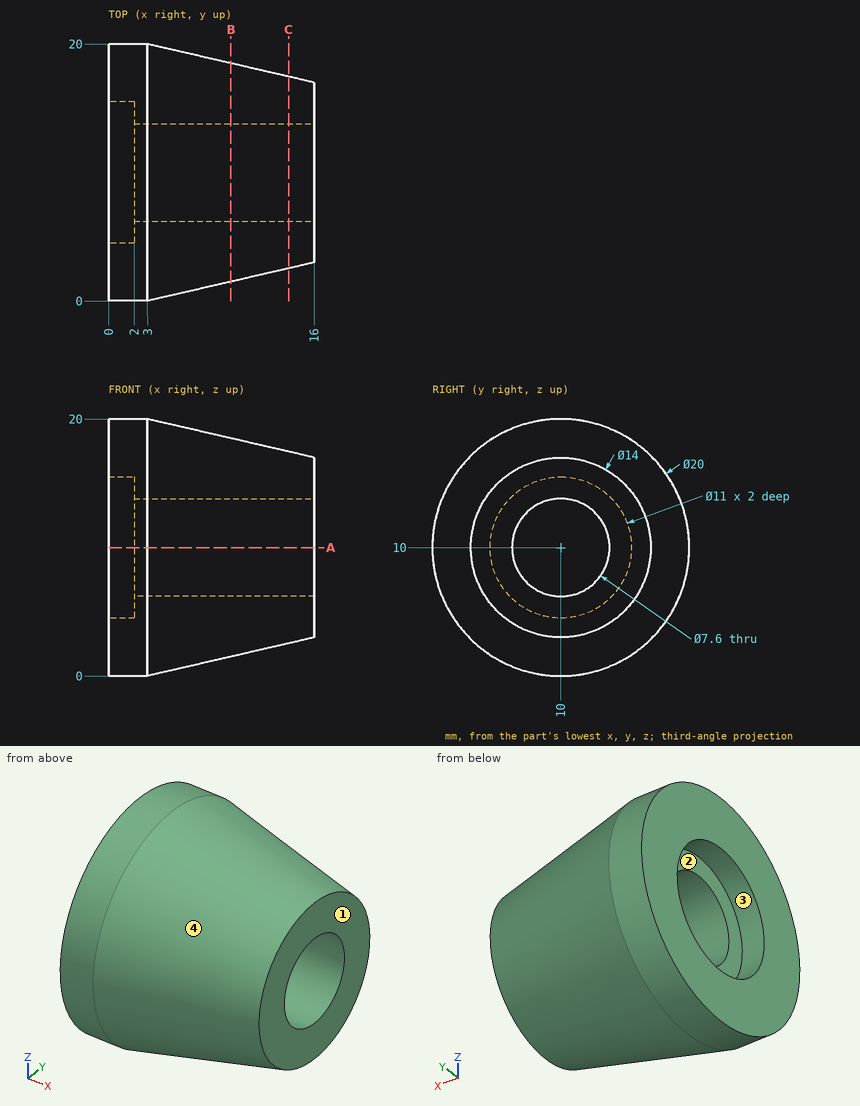
Geometry check sheet. Reference: drawing and pictorial views, mm from the part's lowest x, y, z. Give positions to 0.01 mm unless a question says otherwise; leave off trailing zeros. Write each loop counter-clockwise with the first axis right and the second up, starting at its lowest first coordinate (ties: lowest second). Pieces come first, ordered by that corner, then holes. Notation, with made-up numbers: M -8,58 L 24,58 A23 cw 24,78 Z; hole C 29.5,76.5 d5. An arc over 180 degrees is marked long. Answer as CSV lines item,"result". Start each with the question number.
Q1. Release check for a two-part mould opening along Y. For the marked faces 1, 2, 3 and 4 record: pulls with the +Y half, pulls with the -Y half, needs draft (parallel to the pull), parting line crosses it, or undercut.
Q2. Section check B-B, the plane x = 9.5. Record the cut outline in (y, z).
Q3. Section check C-C, the plane x = 14. Record the cut outline in (y, z), then the cut area to 3 significant figures.
Q4. Section check A-A, the plane z = 10. Record the cut outline in (x, y), then the cut area to 3 significant figures.
Q5. Material ranges on L1, parallel to Y at x = 1.2, z = 10; L2, parallel to Y at x = 9.25, z = 9.5; L3, parallel to X at y = 6.5, z = 13, recorded low to high.
Q6. Go/stop test with flat-tipped pins: pin 1 (6 mm diameter, centred on x = 4.5, z = 6, fed in from -Y); pin 2 (6 mm diameter, centred on x = 9.5, y = 15, fed in from +Z); pin 3 (1 mm diameter, centred on x = 6, z = 15, fed in from -Y). Record where each tip stops, or that it passes through.
Geometry says:
1,face 1,"needs draft"
1,face 2,"undercut"
1,face 3,"undercut"
1,face 4,"parting line crosses it"
2,outline,"C 10,10 d17; hole C 10,10 d7.6"
3,outline,"C 10,10 d14.92; hole C 10,10 d7.6"
3,area,"130 mm^2"
4,outline,"M 0,0 L 3,0 L 16,3 L 16,6.2 L 2,6.2 L 2,4.5 L 0,4.5 Z; M 0,15.5 L 2,15.5 L 2,13.8 L 16,13.8 L 16,17 L 3,20 L 0,20 Z"
4,area,"153 mm^2"
5,L1,"0 to 4.5, 15.5 to 20"
5,L2,"1.46 to 6.23, 13.77 to 18.54"
5,L3,"2 to 16"
6,pin 1,"y = 0.1"
6,pin 2,"z = 18.53"
6,pin 3,"y = 1.82"
